```python
from build123d import *

# Parameters (mm, degrees)
F2_R     = 2
F4_DEPTH = 50


with BuildPart() as f1:
    # F0 (on Front) → F1 (revolve)
    with BuildSketch(Plane.XZ):
        Polygon((35, 14.7952197132), (0, 14.7952197132), (0, 11.7952197132), (33, 13.7952197132), (15, -15.2047802868), (35, -15.2047802868), align=None)
    revolve(axis=Axis((0, 0, 13.2952197132), (0, 0, -1)))

    # F2
    f2_edges = [f1.edges().sort_by_distance(p)[0] for p in [
        (-35, 0, 14.79522),
    ]]
    fillet(f2_edges, radius=F2_R)

    # F3 (on Front) → F4 (cut)
    with BuildSketch(Plane.XZ):
        with BuildLine():
            Line((-2.5, -12.7047802868), (2.5, -12.7047802868))
            ThreePointArc((2.5, -12.7047802868), (0, -10.2047802868), (-2.5, -12.7047802868))
        make_face()
        with BuildLine():
            Line((2.5, -17.7047802868), (2.5, -12.7047802868))
            ThreePointArc((2.5, -12.7047802868), (0, -15.2047802868), (-2.5, -12.7047802868))
            Line((-2.5, -12.7047802868), (-2.5, -17.7047802868))
            Line((-2.5, -17.7047802868), (2.5, -17.7047802868))
        make_face()
        with BuildLine():
            ThreePointArc((-2.5, -12.7047802868), (0, -15.2047802868), (2.5, -12.7047802868))
            Line((2.5, -12.7047802868), (-2.5, -12.7047802868))
        make_face()
    extrude(amount=-F4_DEPTH, mode=Mode.SUBTRACT)


solid = f1.part
```
Design review of the part built by this model. Coordinates are the model's own, in mm. A direction names the side the tool comes from. Give positions to 0.01 mm unless a question says otherwise; leave off trailing zeros. Order: outer loops, then holes, each group sorted by start corner. A loop starts at its lowest first (then second) coordinate and runs counter-clockwise, first axis right, second up. Notation, with made-up numbers: M -34.75,37.5 L 0.25,37.5 A31 cw 0.25,69.5 Z; hole C 40,89 d10. An arc over 180 degrees is marked long. One line per question, with ' | ' between items. Start each with the question number.
Q1. Machinability: for faces 5 (the face through (0.055, 25.552, -10.205)), 6 (the face through (0, 0, 14.795)), which of the approach directions +Z, -Z, +X, -X, +Y, -Y give a long, thin tool a straight path to every point of the face, cutting with its end or side? Answer none if there is none.
Q2. We need section A-A (z = 0). Write out the cut boundary in (x, y), plus the area to 3 significant figures.
Q3. For L1, parallel to Z at x = 2.5, y = -20; L2, parallel to X at y = -4.5, z = 9; L3, parallel to Y at x = 12, z = -2, list the stretches that pass through material, from the lowest coordinate up. Write a range as [from, to].
Q4. The part is to be moulded in two halves that separate along Y. For faces 1 (the face through (-2.5, 25, -14)), 2 (the face through (-0.45, 2.02, 11.92)), 3 (the face through (-14.184, 10.876, -10.574)), 4 (the face through (-28, 21, -1)), say which applies: +Y half, -Y half, draft (parallel to the pull), parting line (faces both ways), or undercut.
Q5. For pin 1 Ø1 at (y, z) = (-13, -11) entering from +X; pin 2 Ø6 at (x, z) = (-24.5, 0) entering from +Y; pin 3 Ø6 at (y, z) = (-9.5, 2) entering from +X, all flat-tipped, find the tip position at first contact; note any pin that passes through.
Q6. We need section B-B (z = 4.5). Write out the cut boundary in (x, y), plus the area to 3 significant figures.
Returned:
1) face 5: -Z, +Y | face 6: +Z, +X, -X, +Y, -Y
2) outline: C 0,0 d70; hole C 0,0 d48.87 | area: 1,970 mm2
3) L1: [-15.2, -6.9], [13.02, 14.8] | L2: [-34.71, -29.68], [29.68, 34.71] | L3: [-32.88, -19.85], [19.85, 32.88]
4) face 1: draft | face 2: undercut | face 3: undercut | face 4: parting line
5) pin 1: x = 32.69 | pin 2: y = 27.62 | pin 3: x = 34.39
6) outline: C 0,0 d70; hole C 0,0 d54.46 | area: 1,520 mm2
